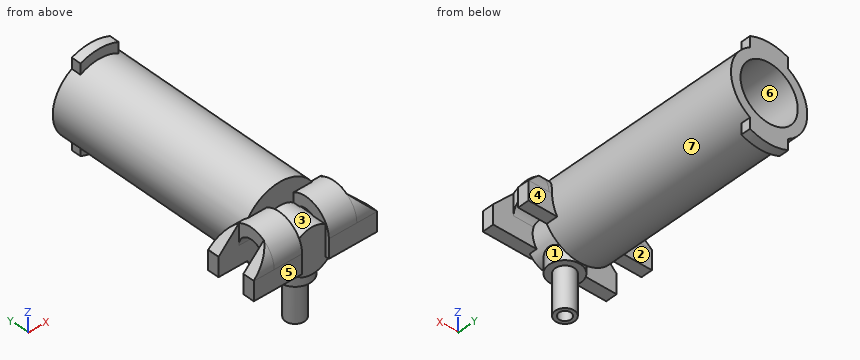
```python
from build123d import *
from build123d.topology import SkipClean

# Parameters (mm, degrees)
SKETCH1_R            = 6
BOSS_EXTRUDE1_DEPTH  = 32.7
SHELL1_T             = -1.5
SKETCH2_R            = 3.5
BOSS_EXTRUDE3_DEPTH  = 5.5
SHELL3_START         = -4
SHELL3_OUTLINE_R     = 2
SHELL3_DEPTH         = 5.5
SKETCH4_R            = 2.5
BOSS_EXTRUDE4_DEPTH  = 6.1
SKETCH7_R            = 1.5
BOSS_EXTRUDE6_DEPTH  = 6.3
SKETCH8_R            = 0.95
CUT_EXTRUDE1_DEPTH   = 12.3
SKETCH9_R            = 2
CUT_EXTRUDE2_DEPTH   = 40.200127551
BOSS_EXTRUDE7_DEPTH  = 6.5
SKETCH11_W           = 2.1
SKETCH11_H           = 4.759411023
CUT_EXTRUDE3_DEPTH   = 41.684763873
CUT_EXTRUDE4_DEPTH   = 36.571055794
SKETCH13_W           = 4.4
SKETCH13_H           = 1.797977648
BOSS_EXTRUDE8_DEPTH  = 3
SKETCH15_W           = 4.39606385
SKETCH15_H           = 1.797977648
BOSS_EXTRUDE9_DEPTH  = 3
SKETCH16_R           = 2
CUT_EXTRUDE5_DEPTH   = 40.279765925
SKETCH17_R           = 4.5
CUT_EXTRUDE6_DEPTH   = 35.197222256
SKETCH18_W           = 3.024802645
SKETCH18_H           = 1.797977648
BOSS_EXTRUDE10_DEPTH = 3.2
BOSS_EXTRUDE11_DEPTH = 1.797977648
CUT_EXTRUDE11_DEPTH  = 38.138928519
BOSS_EXTRUDE12_DEPTH = 1.797977648
CUT_EXTRUDE12_DEPTH  = 38.138928519
BOSS_EXTRUDE13_START = -1.5
BOSS_EXTRUDE13_DEPTH = 1.5


# Read off the part's stored shape, not the designer's step: Shell3
with BuildPart() as part:
    # Sketch1 → Boss-Extrude1 (new body)
    with BuildSketch(Plane(origin=(0, 0, 0), x_dir=(1, 0, 0), z_dir=(0, 1, 0))):
        with Locations(Location((0, 0, 0), (0, 0, 270))):
            Circle(SKETCH1_R)
    extrude(amount=BOSS_EXTRUDE1_DEPTH)

    # Shell1
    shell1_openings = [part.faces().sort_by_distance(p)[0] for p in [
        (0, 32.7, 0),
    ]]
    offset(amount=SHELL1_T, openings=shell1_openings, kind=Kind.INTERSECTION)

    # Sketch2 → Boss-Extrude3 (add)
    with BuildSketch(Plane.XZ):
        with Locations(Location((0, -1, 0), (0, 0, 270))):
            Circle(SKETCH2_R)
    extrude(amount=BOSS_EXTRUDE3_DEPTH)

    # Shell3 outline → Shell3 (cut)
    with BuildSketch(Plane(origin=(0, 0, 0), x_dir=(1, 0, 0), z_dir=(0, 1, 0)).offset(SHELL3_START)):
        with Locations((0, 1)):
            Circle(SHELL3_OUTLINE_R)
    extrude(amount=SHELL3_DEPTH, mode=Mode.SUBTRACT)

    # Sketch4 → Boss-Extrude4 (add)
    with BuildSketch(Plane.XY):
        with Locations((0, -2.573540176)):
            Circle(SKETCH4_R)
    extrude(amount=-BOSS_EXTRUDE4_DEPTH)

    # Sketch7 → Boss-Extrude6 (add)
    with BuildSketch(Plane(origin=(0, 0, -6.1), x_dir=(-1, 0, 0), z_dir=(0, 0, -1))):
        with Locations((0, -2.573540176)):
            Circle(SKETCH7_R)
    extrude(amount=BOSS_EXTRUDE6_DEPTH)

    # Sketch8 → Cut-Extrude1 (cut)
    with BuildSketch(Plane(origin=(0, 0, -12.4), x_dir=(-1, 0, 0), z_dir=(0, 0, -1))):
        with Locations((0, -2.573540176)):
            Circle(SKETCH8_R)
    extrude(amount=-CUT_EXTRUDE1_DEPTH, mode=Mode.SUBTRACT)

    # Sketch9 → Cut-Extrude2 (cut, through all)
    with BuildSketch(Plane(origin=(0, -4, 0), x_dir=(1, 0, 0), z_dir=(0, 1, 0))):
        with Locations(Location((0, 1, 0), (0, 0, 270))):
            Circle(SKETCH9_R)
    extrude(amount=CUT_EXTRUDE2_DEPTH, mode=Mode.SUBTRACT)

    # Sketch10 → Boss-Extrude7 (add)
    with BuildSketch(Plane(origin=(0, 0, 0), x_dir=(0, 0, -1), z_dir=(1, 0, 0))):
        with BuildLine():
            Line((0, -4.3), (0, -6.097977648))
            ThreePointArc((0, -6.097977648), (-3.947977648, -2.15), (0, 1.797977648))
            Line((0, 1.797977648), (0, 0))
            ThreePointArc((0, 0), (-2.15, -2.15), (0, -4.3))
        make_face()
    extrude(amount=BOSS_EXTRUDE7_DEPTH)

    # Sketch11 → Cut-Extrude3 (cut, through all)
    with BuildSketch(Plane.XZ.offset(5.5)):
        with Locations((1.05, 2.379705512)):
            Rectangle(SKETCH11_W, SKETCH11_H)
    extrude(amount=CUT_EXTRUDE3_DEPTH, mode=Mode.SUBTRACT)

    # Sketch12 → Cut-Extrude4 (cut, through all)
    with BuildSketch(Plane.XZ):
        with BuildLine():
            Line((2.105734518, 1.795689922), (2.105734518, 3.947977648))
            Line((2.105734518, 3.947977648), (0, 3.947977648))
            Line((0, 3.947977648), (0, 2.5))
            ThreePointArc((0, 2.5), (1.110199368, 2.319255544), (2.105734518, 1.795689922))
        make_face()
    extrude(amount=CUT_EXTRUDE4_DEPTH, mode=Mode.SUBTRACT)

    # Sketch13 → Boss-Extrude8 (add)
    with BuildSketch(Plane(origin=(0, 0, 0), x_dir=(-1, 0, 0), z_dir=(0, 0, -1))):
        with Locations((-4.3, -5.198988824)):
            Rectangle(SKETCH13_W, SKETCH13_H)
    extrude(amount=BOSS_EXTRUDE8_DEPTH)

    # Sketch15 → Boss-Extrude9 (add)
    with SkipClean():  # the faces are left unmerged after this step: merging them gives an invalid solid
        with BuildSketch(Plane(origin=(0, 0, 0), x_dir=(-1, 0, 0), z_dir=(0, 0, -1))):
            with Locations((-4.301968075, 0.898988824)):
                Rectangle(SKETCH15_W, SKETCH15_H)
        extrude(amount=BOSS_EXTRUDE9_DEPTH)

    # Sketch16 → Cut-Extrude5 (cut, through all)
    with SkipClean():  # the faces are left unmerged after this step: merging them gives an invalid solid
        with BuildSketch(Plane(origin=(0, -4, 0), x_dir=(1, 0, 0), z_dir=(0, 1, 0))):
            with Locations(Location((0, 1, 0), (0, 0, 270))):
                Circle(SKETCH16_R)
        extrude(amount=CUT_EXTRUDE5_DEPTH, mode=Mode.SUBTRACT)

    # Sketch17 → Cut-Extrude6 (cut, through all)
    with SkipClean():  # the faces are left unmerged after this step: merging them gives an invalid solid
        with BuildSketch(Plane(origin=(0, 1.5, 0), x_dir=(1, 0, 0), z_dir=(0, 1, 0))):
            with Locations(Location((0, 0, 0), (0, 0, 270))):
                Circle(SKETCH17_R)
        extrude(amount=CUT_EXTRUDE6_DEPTH, mode=Mode.SUBTRACT)

    # Sketch18 → Boss-Extrude10 (add)
    with SkipClean():  # the faces are left unmerged after this step: merging them gives an invalid solid
        with BuildSketch(Plane(origin=(6.5, 0, 0), x_dir=(0, 0, -1), z_dir=(1, 0, 0))):
            with Locations((1.487598678, 0.898988824)):
                Rectangle(SKETCH18_W, SKETCH18_H)
            with Locations((1.487598678, -5.198988824)):
                Rectangle(SKETCH18_W, SKETCH18_H)
        extrude(amount=BOSS_EXTRUDE10_DEPTH)

    # Sketch19 → Boss-Extrude11 (add)
    with SkipClean():  # the faces are left unmerged after this step: merging them gives an invalid solid
        with BuildSketch(Plane(origin=(0, -4.3, 0), x_dir=(1, 0, 0), z_dir=(0, 1, 0))):
            Polygon((6.5, -3.285642739), (6.5, 0), (9.7, -0.024802645), align=None)
        extrude(amount=-BOSS_EXTRUDE11_DEPTH)

    # Sketch22 → Cut-Extrude11 (cut, through all)
    with SkipClean():  # the faces are left unmerged after this step: merging them gives an invalid solid
        with BuildSketch(Plane.ZY.offset(-6.5)):
            with BuildLine():
                Line((0, -6.097977648), (3.285642739, -6.097977648))
                Line((3.285642739, -6.097977648), (3.285642739, -4.33885342))
                ThreePointArc((3.285642739, -4.33885342), (1.863462252, -5.630522366), (0, -6.097977648))
            make_face()
        extrude(amount=-CUT_EXTRUDE11_DEPTH, mode=Mode.SUBTRACT)

    # Sketch24 → Boss-Extrude12 (add)
    with SkipClean():  # the faces are left unmerged after this step: merging them gives an invalid solid
        with BuildSketch(Plane.XZ):
            Polygon((9.7, 0), (6.5, 3.285642739), (6.5, 0.012401323), align=None)
        extrude(amount=-BOSS_EXTRUDE12_DEPTH)

    # Sketch25 → Cut-Extrude12 (cut, through all)
    with SkipClean():  # the faces are left unmerged after this step: merging them gives an invalid solid
        with BuildSketch(Plane.ZY.offset(-6.5)):
            with BuildLine():
                Line((3.285642739, 0.03885342), (3.285642739, 1.797977648))
                Line((3.285642739, 1.797977648), (0, 1.797977648))
                ThreePointArc((0, 1.797977648), (1.863462252, 1.330522366), (3.285642739, 0.03885342))
            make_face()
        extrude(amount=-CUT_EXTRUDE12_DEPTH, mode=Mode.SUBTRACT)

    # Mirror3: part across plane


with BuildPart() as part_1:
    add(part.part)
    add(part.part.mirror(Plane(origin=(0, 0, 0), x_dir=(0, 0, 1), z_dir=(1, 0, 0))))

    # Sketch26 → Boss-Extrude13 (add)
    with SkipClean():  # the faces are left unmerged after this step: merging them gives an invalid solid
        with BuildSketch(Plane(origin=(0, 32.7, 0), x_dir=(1, 0, 0), z_dir=(0, 1, 0)).offset(BOSS_EXTRUDE13_START)):
            with BuildLine():
                Line((3, 5.196152423), (3, 6.873863542))
                ThreePointArc((3, 6.873863542), (0, 7.5), (-3, 6.873863542))
                Line((-3, 6.873863542), (-3, 5.196152423))
                ThreePointArc((-3, 5.196152423), (0, 6), (3, 5.196152423))
            make_face()
            with BuildLine():
                Line((3, -5.196152423), (3, -6.873863542))
                ThreePointArc((3, -6.873863542), (0, -7.5), (-3, -6.873863542))
                Line((-3, -6.873863542), (-3, -5.196152423))
                ThreePointArc((-3, -5.196152423), (0, -6), (3, -5.196152423))
            make_face()
        extrude(amount=BOSS_EXTRUDE13_DEPTH)


solid = part_1.part
```
CAD build for the part. Positions are in the model's coordinates, mm. Face numbers are marked on the shaded views. A direction names the side the tool comes from. Round coordinates to 2 decimals unless told otherwise and drop trailing zeros. Order: outer loops, then holes, each group sorted by start corner. A loop starts at its lowest first (then second) coordinate and runs counter-clockwise, first axis right, second up.
Item 1: Pin check, flat tips, straight feed: pin 1 (0.8 mm diameter, centred on y = 31.5, z = -6, fed in from -X); pin 2 (5 mm diameter, centred on y = 26.5, z = 4.5, fed in from +X); pin 3 (1.4 mm diameter, centred on x = 6.5, y = -5, fed in from -Z). Stop position of each tip, or through.
Item 2: Saw through at A-A on x = 8. Write the cut outline in (y, z), then the cut area to 3 significant figures.
Item 3: Tool access for the marked faces 1, 2, 3 and 4: list every direction of +Z, -Z, +X, -X, +Y, -Y with a clear straight run to the whole face (end or side of a thin tool).
Item 4: Saw through at B-B on y = -2.15. Write the cut outline in (x, z), then the cut area to 3 significant figures.
Item 5: Mould opens along Z. For the marked faces 5, 6 and 7 say: pulls with the +Z half, pulls with the -Z half, needs draft (parallel to the pull), parting line crosses it, or undercut.
Item 6: Saw through at C-C on y = 29.5. Write the cut outline in (x, z), then the cut area to 3 significant figures.
Item 7: Saw through at D-D on x = -7.5. Write the cut outline in (y, z).
Item 8: Probe line 1 along Z through (x, y) = (0, 10.5); line 2 along Y through (x, z) = (-7, -2.75); line 3 along X through (y, z) = (-2.4, -1). List the from-to ranges inside material, lowest first.
Reported:
1. pin 1: stops at x = -3
1. pin 2: stops at x = 5.66
1. pin 3: stops at z = -3
2. outline: (-6.1, -3) - (-4.3, -3) - (-4.3, 1.76) - (-5.69, 1.76) arc R3.95 ccw to (-6.1, 0) - close; (0, -3) - (1.8, -3) - (1.8, 0) arc R3.95 ccw to (1.39, 1.75) - (0, 1.75) - close
2. area: 16.6 mm2
3. face 1: -Z
3. face 2: -Z, -X, +Y
3. face 3: none
3. face 4: -Z, +X, +Y
4. outline: (-6.5, 2.15) - (-2.11, 2.15) - (-2.11, 3.95) - (-6.5, 3.95) - close; (-2.46, -6.1) - (-1.44, -6.1) - (-1.44, -12.4) - (-0.85, -12.4) - (-0.85, -2.81) arc R2 cw (long way) to (0.85, -2.81) - (0.85, -12.4) - (1.44, -12.4) - (1.44, -6.1) - (2.46, -6.1) - (2.46, -3.49) arc R3.5 ccw (long way) to (-2.46, -3.49) - close; (2.11, 2.15) - (6.5, 2.15) - (6.5, 3.95) - (2.11, 3.95) - close
4. area: 53.2 mm2
5. face 5: needs draft
5. face 6: undercut
5. face 7: parting line crosses it
6. outline: circle Ø12 at (0, 0); hole circle Ø9 at (0, 0)
6. area: 49.5 mm2
7. outline: (-6.1, -3) - (-4.3, -3) - (-4.3, 2.27) - (-5.38, 2.27) arc R3.95 ccw to (-6.1, 0) - close; (0, -3) - (1.8, -3) - (1.8, 0) arc R3.95 ccw to (1.09, 2.26) - (0, 2.26) - close
8. line 1: z = -6 to -4.5, 4.5 to 6
8. line 2: y = -6.1 to -4.3, 0 to 1.8
8. line 3: x = -3.5 to -2, 2 to 3.5
